Part model, mm, in its own coordinate system. A direction names the side the tool comes from. Coordinates: 2 decimals unless noted, no trailing zeros. Order: outer loops, then holes, each group sorted by start corner. A loop starts at its lowest first (then second) coordinate and runs counter-clockwise, first axis right, second up.
Autodesk Inventor part; units mm, degrees
ref_plane "YZ Plane" through (0, 0, 0) normal (1, 0, 0) x (0, 1, 0)
ref_plane "XZ Plane" through (0, 0, 0) normal (0, 1, 0) x (-1, 0, 0)
ref_plane "XY Plane" through (0, 0, 0) normal (0, 0, 1) x (1, 0, 0)
sketch "Sketch1" plane through (0, 0, 0) normal (0, 1, 0) x (-1, 0, 0)
  line L0 (0, 0) -> (76.2, 0)
  line L1 (76.2, 0) -> (76.2, -50.8)
  line L2 (76.2, -50.8) -> (0, -50.8)
  line L3 (0, -50.8) -> (0, 0)
  dimension "d0" = 76.2
  dimension "d1" = 50.8
extrude "Extrusion1" add sketch "Sketch1" along normal blind 6.35
sketch "Sketch2" plane through (0, 6.35, 0) normal (0, 1, 0) x (1, 0, 0)
  line L0 (0, 0) -> (0, 50.8)
  line L1 (-76.2, 50.8) -> (-76.2, 0)
  line L2 (0, 50.8) -> (-76.2, 0)
  line L3 (-76.2, 0) -> (-76.2, 50.8)
  line L4 (-76.2, 50.8) -> (0, 0)
  circle A0 centre (-38.1, 25.4) radius 14.2875
  dimension "d4" = 28.575
hole "Hole1" at (-38.1, 6.35, -25.4) direction (0, -1, 0) diameter 28.575 end through all
sketch "Sketch3" plane through (0, 6.35, 0) normal (0, 1, 0) x (1, 0, 0)
  line L0 (0, 50.8) -> (0, 0)
  line L1 (0, 25.4) -> (-23.8125, 25.4)
  circle A0 centre (-38.1, 25.4) radius 14.2875
  line L2 (-52.3875, 25.4) -> (-76.2, 25.4) construction
  line L3 (-76.2, 0) -> (-76.2, 50.8)
  line L4 (-69.0563, 25.4) -> (-59.5312, 25.4) construction
  line L5 (-69.0563, 22.606) -> (-59.5312, 22.606)
  line L6 (-59.5312, 28.194) -> (-69.0563, 28.194)
  arc A1 (-69.0563, 28.194) -> (-69.0563, 22.606) centre (-69.0563, 25.4) ccw
  arc A2 (-59.5312, 22.606) -> (-59.5312, 28.194) centre (-59.5312, 25.4) ccw
  line L7 (-16.6688, 25.4) -> (-7.1437, 25.4) construction
  line L8 (-16.6688, 22.606) -> (-7.1437, 22.606)
  line L9 (-7.1437, 28.194) -> (-16.6688, 28.194)
  arc A3 (-16.6688, 28.194) -> (-16.6688, 22.606) centre (-16.6688, 25.4) ccw
  arc A4 (-7.1437, 22.606) -> (-7.1437, 28.194) centre (-7.1437, 25.4) ccw
  point P0 (-64.2938, 25.4)
  point P1 (-11.9062, 25.4)
  dimension "d12" = 4.7625
  dimension "d13" = 5.588
  dimension "d14" = 4.7625
  dimension "d15" = 5.588
extrude "Extrusion2" cut sketch "Sketch3" against normal blind 6.35 contours A4 L8 A3 L1 | L1 A3 L9 A4 | A1 L6 A2 L5
sketch "Sketch4" plane through (0, 6.35, 0) normal (0, 1, 0) x (1, 0, 0)
  point P0 (0, 0)
sketch "Sketch5" plane through (0, 6.35, 0) normal (0, 1, 0) x (1, 0, 0)
  line L0 (0, 0) -> (0, 50.8)
  line L1 (0, 0) -> (0, 15.24)
  line L2 (0, 15.24) -> (-20.32, 15.24)
  line L3 (-20.32, 15.24) -> (-20.32, 0)
  line L4 (0, 50.8) -> (-20.32, 50.8)
  line L5 (-20.32, 50.8) -> (-20.32, 35.56)
  line L6 (-20.32, 35.56) -> (0, 35.56)
  line L7 (0, 35.56) -> (0, 50.8)
  line L8 (0, 50.8) -> (-76.2, 50.8)
  line L9 (-76.2, 50.8) -> (-76.2, 35.56)
  line L10 (-76.2, 50.8) -> (-76.2, 0)
  line L11 (-76.2, 0) -> (0, 0)
  line L12 (-76.2, 0) -> (-76.2, 15.24)
  line L13 (-76.2, 15.24) -> (-55.88, 15.24)
  line L14 (-55.88, 15.24) -> (-55.88, 0)
  line L15 (-76.2, 35.56) -> (-55.88, 35.56)
  line L16 (-55.88, 35.56) -> (-55.88, 50.8)
  line L17 (-76.2, 0) -> (-55.88, 0)
  line L18 (-76.2, 15.24) -> (-55.88, 15.24)
  line L19 (-20.32, 0) -> (0, 0)
  line L20 (-55.88, 50.8) -> (-76.2, 50.8)
  dimension "d19" = 15.24
  dimension "d20" = 20.32
  dimension "d21" = 20.32
  dimension "d22" = 15.24
  dimension "d23" = 20.32
extrude "Extrusion3" cut sketch "Sketch5" against normal blind 25.4 contours L11 L3 L2 L0 | L6 L5 L4 L0 | L11 L10 L13 L14 | L16 L15 L9 L8
fillet "Fillet2" radius 3.175 8 edges at (-55.88, 3.175, -50.8) (-76.2, 3.175, -35.56) (-76.2, 3.175, -15.24) (-55.88, 3.175, 0) (0, 3.175, -15.24) (0, 3.175, -35.56) (-20.32, 3.175, -50.8) (-20.32, 3.175, 0)
fillet "Fillet3" radius 11.1125 4 edges at (-20.32, 3.175, -35.56) (-55.88, 3.175, -35.56) (-55.88, 3.175, -15.24) (-20.32, 3.175, -15.24)
properties part number "4461-17-0101 Tensioner Plate" material "Aluminum 6061"
Q1. Cut at D-D on x = -11.5. Write the cut outline in (y, z).
Results list:
outline: (0, -35.8) - (6.35, -35.8) - (6.35, -28.19) - (0, -28.19) - close; (0, -22.61) - (6.35, -22.61) - (6.35, -15) - (0, -15) - close
Q2. Wall check: line 1 along X through (y, z) = (3.25, -25.4); line 2 along Z through (x, y) = (-38.1, 3.5); line 3 along Z through (x, y) = (-7.5, 0.5). Give the ranges that are in metal, low to high.
Results list:
line 1: x = -76.2 to -71.85, -56.74 to -52.39, -23.81 to -19.46, -4.35 to 0
line 2: z = -50.8 to -39.69, -11.11 to 0
line 3: z = -35.56 to -28.19, -22.61 to -15.24
Q3. Cut at B-B on z = -25.4. Write the cut outline in (x, y), and give its area (3 significant figures).
Results list:
outline: (-76.2, 0) - (-71.85, 0) - (-71.85, 6.35) - (-76.2, 6.35) - close; (-56.74, 0) - (-52.39, 0) - (-52.39, 6.35) - (-56.74, 6.35) - close; (-23.81, 0) - (-19.46, 0) - (-19.46, 6.35) - (-23.81, 6.35) - close; (-4.35, 0) - (0, 0) - (0, 6.35) - (-4.35, 6.35) - close
area: 110 mm2
Q4. Cut at A-A on x = -32. Write the cut outline in (y, z), and give its area (3 significant figures).
Results list:
outline: (0, -50.8) - (6.35, -50.8) - (6.35, -38.32) - (0, -38.32) - close; (0, -12.48) - (6.35, -12.48) - (6.35, 0) - (0, 0) - close
area: 158 mm2
Q5. Which spindle directions (+Z, -Z, +X, -X, +Y, -Y) get a long thin tool onto all of the face, cutting with end or side? Do faces 1 (the face through (-70, 3, -35.56)), 2 (the face through (-76.2, 3, -25)), 3 (the face through (-4.35, 3.22, -25.34)). Say none if no direction does.
Results list:
face 1: -Z, -X, +Y, -Y
face 2: +Z, -Z, -X, +Y, -Y
face 3: +Y, -Y
Q6. Mould opens along Z. For faces 4 (the face through (-59.05, 3.13, -38.9)), 5 (the face through (-64, 3, -28.194)), 6 (the face through (-56.738, 3.219, -25.339)), 7 (the face through (-70, 3, -15.24)) say: pulls with the +Z half, pulls with the -Z half, needs draft (parallel to the pull), parting line crosses it, or undercut.
Results list:
face 4: pulls with the -Z half
face 5: undercut
face 6: undercut
face 7: pulls with the +Z half
Q7. Pin check, flat tips, straight feed: pin 1 Ø3 at (x, y) = (-64, 2) entering from -Z; pin 2 Ø1.5 at (x, z) = (-68.5, -15) entering from -Y; pin 3 Ø3 at (x, y) = (-6.5, 4) entering from -Z; pin 4 Ø1.9 at (x, y) = (-14, 2) entering from -Z. Stop position of each tip, or through.
Results list:
pin 1: stops at z = -36.51
pin 2: stops at y = 0
pin 3: stops at z = -35.56
pin 4: stops at z = -37.16
Q8. Cut at C-C on y = 4.25. Count the separate pieces of the cut face and the enclosed holes in it, and give its area (3 significant figures).
Results list:
separate pieces: 1
enclosed holes: 3
area: 1,920 mm2
